Geometry check sheet. Reference: the model listing, model coordinates, mm. Face numbers are marked on the shaded views. A direction names the side the tool comes from. Give positions to 0.01 mm unless a question says otherwise; leave off trailing zeros. Loops run counter-clockwise (first coordinate to the right, second up) from the corner with the lowest first, then second, coordinate; pieces in that order, holes last. Notation, with made-up numbers: (-20.75, 18) -> (19.25, 18) arc R26 cw to (19.25, 54) -> close; hole circle Ø2 at (-34.5, 14.5). An arc over 180 degrees is marked (long way). Write each question's results on one line, items separated by ' | '. Start each with the question number.
1) Sectioned sample at B-B on z = -38.5. Record the cut outline in (x, y), then the cut area to 3 significant figures.
2) Sectioned sample at A-A on x = 4.85. Count the separate pieces of the cut face and the enclosed holes in it, then the cut area to 3 significant figures.
3) Depth check by flat-ended pin: pin 1 (1.5 mm diameter, centred on x = 3.5, y = 49.5, fed in from -Z); pin 2 (0.9 mm diameter, centred on x = 1.5, y = 35, fed in from -Z); pin 3 (2 mm diameter, centred on y = 36.5, z = -28.5, fed in from -X). Enter the tip coordinate at first touch or a pass-through.
4) Scan lines: line 1 (Z direction, x = 3.6, y = 43); line 2 (Y direction, x = 4.2, z = -23); line 3 (Z direction, x = 1.2, y = 39). Record each from-to range of solid material in increasing order. Write a range as from..to.
5) Sectioned sample at C-C on x = 1.35. Record the cut outline in (y, z), then the cut area to 3 significant figures.
6) Set-up check for the marked faces 1, 2 and 3: record each of +Z, -Z, +X, -X, +Y, -Y from which the full face is reachable in a straight line by a thin tool's end or side.
7) Draft check along Z on the marked faces 4, 5 and 6. Enter one of: pulls with the +Z half, pulls with the -Z half, needs draft (parallel to the pull), parting line crosses it, or undercut.
```python
from build123d import *

# Parameters (mm, degrees)
SKETCH27_R          = 3.55
SKETCH27_R_2        = 4
SKETCH27_R_3        = 2.5
SKETCH27_R_4        = 1.5
BOSS_EXTRUDE1_DEPTH = 6
SKETCH47_R          = 4.99
CUT_EXTRUDE8_DEPTH  = 3
CUT_EXTRUDE10_DEPTH = 3.5
SKETCH49_W          = 24
SKETCH49_H          = 6
CUT_EXTRUDE11_DEPTH = 3
SKETCH50_R          = 1.5
CUT_EXTRUDE12_DEPTH = 3
FILLET1_R           = 3
CUT_EXTRUDE13_REACH = 5
SKETCH51_R          = 1.5
FILLET2_R           = 10
FILLET3_R           = 2


with BuildPart() as part:
    # Sketch27 → Boss-Extrude1 (new body)
    with BuildSketch(Plane(origin=(0, 0, 0), x_dir=(0, 0, -1), z_dir=(1, 0, 0))):
        with BuildLine():
            Line((4.589716929, 48.674533934), (19.924994259, 58.807513206))
            ThreePointArc((19.924994259, 58.807513206), (31.222626062, 60.983884909), (40.738603868, 54.517104832))
            ThreePointArc((40.738603868, 54.517104832), (44.34906679, 51.201450356), (49.101489768, 50))
            Line((49.101489768, 50), (66, 50))
            Line((66, 50), (66, 45))
            Line((66, 45), (48.564398788, 34))
            Line((48.564398788, 34), (9, 34))
            ThreePointArc((9, 34), (1.33852914, 39.697422256), (4.589716929, 48.674533934))
        make_face()
        with Locations((30.931712199, 54)):
            Circle(SKETCH27_R, mode=Mode.SUBTRACT)
        with Locations((9, 42)):
            Circle(SKETCH27_R_2, mode=Mode.SUBTRACT)
        with Locations((50, 42)):
            Circle(SKETCH27_R_3, mode=Mode.SUBTRACT)
        with Locations((38.919099476, 51.092828782)):
            Circle(SKETCH27_R_4, mode=Mode.SUBTRACT)
        with Locations((22.944324923, 56.907171218)):
            Circle(SKETCH27_R_4, mode=Mode.SUBTRACT)
    extrude(amount=BOSS_EXTRUDE1_DEPTH)

    # Sketch47 → Cut-Extrude8 (cut)
    with BuildSketch(Plane.ZY):
        with Locations((-9, 42)):
            Circle(SKETCH47_R)
    extrude(amount=-CUT_EXTRUDE8_DEPTH, mode=Mode.SUBTRACT)

    # Sketch48 → Cut-Extrude10 (cut)
    with BuildSketch(Plane.ZY):
        with BuildLine():
            Line((-45.322401917, 50.741571677), (-29.852897284, 65.367501227))
            Line((-29.852897284, 65.367501227), (-16.092106493, 56.274883933))
            ThreePointArc((-16.092106493, 56.274883933), (-17.677203396, 56.31769628), (-18.415049974, 54.914148092))
            ThreePointArc((-18.415049974, 54.914148092), (-28.514928411, 41.684901295), (-42.865524712, 50.115850296))
            ThreePointArc((-42.865524712, 50.115850296), (-43.921672049, 51.10520774), (-45.322401917, 50.741571677))
        make_face()
    extrude(amount=-CUT_EXTRUDE10_DEPTH, mode=Mode.SUBTRACT)

    # Sketch49 → Cut-Extrude11 (cut)
    with BuildSketch(Plane.ZY):
        with Locations((-32, 37)):
            Rectangle(SKETCH49_W, SKETCH49_H)
    extrude(amount=-CUT_EXTRUDE11_DEPTH, mode=Mode.SUBTRACT)

    # Sketch50 → Cut-Extrude12 (cut)
    with BuildSketch(Plane.ZY):
        with Locations((-43, 39)):
            Circle(SKETCH50_R)
        with Locations((-21, 39)):
            Circle(SKETCH50_R)
    extrude(amount=-CUT_EXTRUDE12_DEPTH, mode=Mode.SUBTRACT)

    # Fillet1
    fillet1_edges = [part.edges().sort_by_distance(p)[0] for p in [
        (1.5, 37.881966011, -44),
        (1.5, 40, -41.881966011),
        (1.5, 40, -22.118033989),
        (1.5, 37.881966011, -20),
    ]]
    fillet(fillet1_edges, radius=FILLET1_R)

    # Sketch51 → Cut-Extrude13 (cut, up to next)
    with BuildSketch(Plane.ZY.offset(-3), mode=Mode.PRIVATE) as cut_extrude13_sk1:
        with Locations((-41, 37)):
            Circle(SKETCH51_R)
    cut_extrude13_tool1 = extrude(cut_extrude13_sk1.sketch, amount=-CUT_EXTRUDE13_REACH, mode=Mode.PRIVATE) & part.part
    add(cut_extrude13_tool1.solids().sort_by_distance((3, 37, -41))[0], mode=Mode.SUBTRACT)
    # Sketch51 → Cut-Extrude13 (cut, up to next)
    with BuildSketch(Plane.ZY.offset(-3), mode=Mode.PRIVATE) as cut_extrude13_sk2:
        with Locations((-23, 37)):
            Circle(SKETCH51_R)
    cut_extrude13_tool2 = extrude(cut_extrude13_sk2.sketch, amount=-CUT_EXTRUDE13_REACH, mode=Mode.PRIVATE) & part.part
    add(cut_extrude13_tool2.solids().sort_by_distance((3, 37, -23))[0], mode=Mode.SUBTRACT)

    # Fillet2
    fillet2_edges = [part.edges().sort_by_distance(p)[0] for p in [
        (3, 34, -48.564398788),
    ]]
    fillet(fillet2_edges, radius=FILLET2_R)

    # Fillet3
    fillet3_edges = [part.edges().sort_by_distance(p)[0] for p in [
        (3, 50, -66),
        (3, 45, -66),
    ]]
    fillet(fillet3_edges, radius=FILLET3_R)


solid = part.part
```
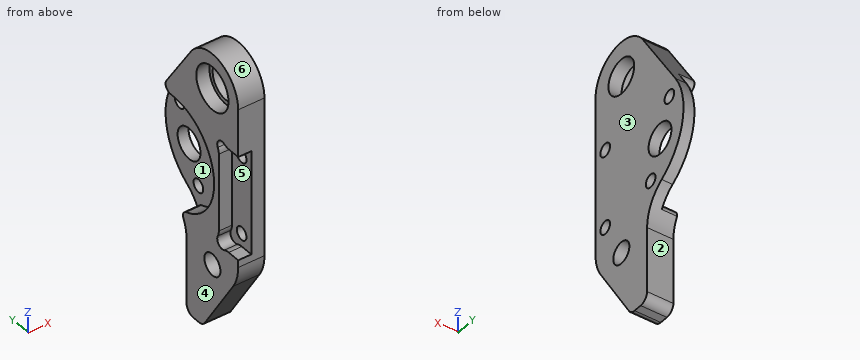
Result:
1) outline: (0, 40) -> (3, 40) -> (3, 34) -> (6, 34) -> (6, 49.65) -> (3.5, 49.65) -> (3.5, 43.99) -> (0, 43.99) -> close; (3.5, 52.53) -> (6, 52.53) -> (6, 57.19) -> (3.5, 57.19) -> close | area: 67.7 mm^2
2) separate pieces: 1 | enclosed holes: 7 | area: 1,050 mm^2
3) pin 1: z = -65.85 | pin 2: z = -50.86 | pin 3: x = 3
4) line 1: -62.83..-52.29, -47.71..-12.87, -5.13..-1.06 | line 2: 34..35.5, 38.5..55.41, 58.41..60.36 | line 3: -56.49..-44.5, -19.5..-12.99, -5.01..-1.58
5) outline: (34, -45.67) arc R10 ccw to (35.54, -51.01) -> (44.41, -65.07) arc R2 ccw to (46.1, -66) -> (48, -66) arc R2 ccw to (50, -64) -> (50, -49.1) arc R10 cw to (51.14, -44.46) arc R1.5 ccw to (50.12, -42.87) arc R12.55 cw to (54.91, -18.42) arc R1.5 ccw to (56.27, -16.09) -> (48.67, -4.59) arc R8 ccw to (34, -9) -> (34, -20) -> (36.94, -20) arc R3 ccw to (38.31, -19.67) arc R1.5 cw to (40.33, -21.69) arc R3 ccw to (40, -23.06) -> (40, -40.94) arc R3 ccw to (40.33, -42.31) arc R1.5 cw to (38.31, -44.33) arc R3 ccw to (36.94, -44) -> (34, -44) -> close; hole circle Ø9.98 at (42, -9); hole circle Ø5 at (42, -50) | area: 570 mm^2
6) face 1: -X, +Y | face 2: -Z, +X, -X, +Y | face 3: +Z, -Z, +X, +Y, -Y
7) face 4: needs draft | face 5: undercut | face 6: pulls with the +Z half
